Check sheet for the modelled part. Datum: model origin and axes. Units: mm. A direction names the side the tool comes from. Coordinates: 2 decimals unless noted, no trailing zeros. Write each loop counter-clockwise with the first axis right and the second up, starting at its lowest first coordinate (ties: lowest second). Pieces come first, ordered by that corner, then holes. Notation, with made-up numbers: M 89.25,73.5 L 140.25,73.5 A19 ccw 140.25,92.5 Z; hole C 34.5,61.5 d2. An arc over 180 degrees is marked long. Answer as CSV lines item,"result".
from build123d import *

# Parameters (mm, degrees)
SKETCH1_W               = 12
SKETCH1_H               = 88.272317903
SKETCH2_W               = 4.5
SKETCH2_H               = 60
CUT_EXTRUDE1_DEPTH      = 13
CUT_EXTRUDE1_DEPTH_BACK = 13
CUT_EXTRUDE2_DEPTH      = 5.5
CUT_EXTRUDE2_DEPTH_BACK = 20.5
SKETCH12_R              = 7.393886086
BOSS_EXTRUDE4_DEPTH     = 15
FILLET2_R               = 40
SKETCH4_R               = 6
CUT_EXTRUDE3_DEPTH      = 6
SKETCH5_R               = 2.25
CUT_EXTRUDE4_DEPTH      = 14.5
SKETCH6_R               = 7.5
BOSS_EXTRUDE1_DEPTH     = 13
SKETCH9_R               = 3.5
SKETCH10_R              = 9
BOSS_EXTRUDE2_DEPTH     = 8
SKETCH11_R              = 3.5
SKETCH11_R_2            = 2.25
BOSS_EXTRUDE3_DEPTH     = 0.5
FILLET1_R               = 0.5
SKETCH13_R              = 12
SKETCH13_R_2            = 3.5
BOSS_EXTRUDE5_DEPTH     = 17
FILLET3_R               = 16
SKETCH16_R              = 77.650275013
CUT_EXTRUDE5_DEPTH      = 22
SKETCH17_R              = 2
CUT_EXTRUDE6_DEPTH      = 22
CUT_EXTRUDE7_START      = -132.272318
SKETCH20_R              = 3.5
CUT_EXTRUDE7_DEPTH      = 132.272318
FILLET5_R               = 1


with BuildPart() as part:
    # Sketch1 → Revolve1 (revolve)
    with BuildSketch(Plane(origin=(0, 0, 0), x_dir=(0, 0, -1), z_dir=(1, 0, 0))):
        with Locations((-6, 44.136158952)):
            Rectangle(SKETCH1_W, SKETCH1_H)
    revolve(axis=Axis((0, 88.272317903, 0), (0, -1, 0)))

    # Sketch2 → Cut-Extrude1 (cut, two sides)
    with BuildSketch(Plane(origin=(0, 0, 0), x_dir=(0, 0, -1), z_dir=(1, 0, 0))) as cut_extrude1_sk:
        with Locations((-9.75, 30)):
            Rectangle(SKETCH2_W, SKETCH2_H)
        with Locations((9.75, 30)):
            Rectangle(SKETCH2_W, SKETCH2_H)
    extrude(amount=CUT_EXTRUDE1_DEPTH, mode=Mode.SUBTRACT)
    extrude(cut_extrude1_sk.sketch, amount=-CUT_EXTRUDE1_DEPTH_BACK, mode=Mode.SUBTRACT)

    # Sketch3 → Cut-Extrude2 (cut, two sides)
    with BuildSketch(Plane.XY.offset(7.5)) as cut_extrude2_sk:
        with BuildLine():
            Line((-12, 40), (-4.905482814, 4.032405892))
            ThreePointArc((-4.905482814, 4.032405892), (0, 0), (4.905482814, 4.032405892))
            Line((4.905482814, 4.032405892), (12, 40))
            Line((12, 40), (12, 0))
            Line((12, 0), (12, -1))
            Line((12, -1), (-12, -1))
            Line((-12, -1), (-12, 0))
            Line((-12, 0), (-12, 40))
        make_face()
    extrude(amount=CUT_EXTRUDE2_DEPTH, mode=Mode.SUBTRACT)
    extrude(cut_extrude2_sk.sketch, amount=-CUT_EXTRUDE2_DEPTH_BACK, mode=Mode.SUBTRACT)

    # Sketch12 → Boss-Extrude4 (add)
    with BuildSketch(Plane.XY.offset(7.5)):
        with Locations((0, 7.393886086)):
            Circle(SKETCH12_R)
    extrude(amount=-BOSS_EXTRUDE4_DEPTH)

    # Fillet2
    fillet2_edges = [part.edges().sort_by_distance(p)[0] for p in [
        (6.324137111, 11.224661628, 0),
        (-6.324137111, 11.224661628, 0),
    ]]
    fillet(fillet2_edges, radius=FILLET2_R)

    # Sketch4 → Cut-Extrude3 (cut)
    with BuildSketch(Plane.XY.offset(7.5)):
        with Locations((0, 5)):
            Circle(SKETCH4_R)
    extrude(amount=-CUT_EXTRUDE3_DEPTH, mode=Mode.SUBTRACT)

    # Sketch5 → Cut-Extrude4 (cut, through all)
    with BuildSketch(Plane.XY.offset(1.5)):
        with Locations((0, 5)):
            Circle(SKETCH5_R)
    extrude(amount=-CUT_EXTRUDE4_DEPTH, mode=Mode.SUBTRACT)

    # Sketch6 → Boss-Extrude1 (add, symmetric)
    with BuildSketch(Plane.XY):
        with Locations((0, 35)):
            Circle(SKETCH6_R)
    extrude(amount=BOSS_EXTRUDE1_DEPTH, both=True)

    # Sketch7 → Cut-Revolve1 (revolve, cut)
    with BuildSketch(Plane(origin=(0, 0, 0), x_dir=(0, 0, -1), z_dir=(1, 0, 0))):
        with BuildLine():
            Line((-7.5, 61.927405715), (-7.5, 51.927405715))
            Line((-7.5, 51.927405715), (-17.5, 51.927405715))
            ThreePointArc((-17.5, 51.927405715), (-24.571067812, 68.998473527), (-7.5, 61.927405715))
        make_face()
        with BuildLine():
            Line((7.5, 51.927405715), (17.5, 51.927405715))
            ThreePointArc((17.5, 51.927405715), (24.571067812, 68.998473527), (7.5, 61.927405715))
            Line((7.5, 61.927405715), (7.5, 51.927405715))
        make_face()
    revolve(axis=Axis((0, 35, 13), (0, 0, -1)), mode=Mode.SUBTRACT)

    # Cut-Sweep1: sweep along a path in Sketch8
    with BuildLine(Plane(origin=(0, 0, 0), x_dir=(0, 0, -1), z_dir=(1, 0, 0))) as cut_sweep1_path:
        Line((0, 88.272317903), (0, 25.420292636))
        ThreePointArc((0, 25.420292636), (3.646414893, 15.617430543), (12.812814028, 10.580608761))
    # Sketch9 → Cut-Sweep1 (sweep, cut)
    with BuildSketch(Plane(origin=(0, 88.272317903, 0), x_dir=(1, 0, 0), z_dir=(0, 1, 0))):
        Circle(SKETCH9_R)
    sweep(path=cut_sweep1_path.line, mode=Mode.SUBTRACT)

    # Sketch10 → Boss-Extrude2 (add, symmetric)
    with BuildSketch(Plane.XY):
        with Locations((0, 35)):
            Circle(SKETCH10_R)
    extrude(amount=BOSS_EXTRUDE2_DEPTH, both=True)

    # Sketch11 → Boss-Extrude3 (add)
    with BuildSketch(Plane.XY.offset(1.5)):
        with Locations((0, 5)):
            Circle(SKETCH11_R)
        with Locations((0, 5)):
            Circle(SKETCH11_R_2, mode=Mode.SUBTRACT)
    extrude(amount=BOSS_EXTRUDE3_DEPTH)

    # Fillet1
    fillet1_edges = [part.edges().sort_by_distance(p)[0] for p in [
        (-5.356920685, 2.297519515, 4.5),
        (5.356920685, 2.297519515, 4.5),
    ]]
    fillet(fillet1_edges, radius=FILLET1_R)

    # Sketch13 → Boss-Extrude5 (add)
    with BuildSketch(Plane(origin=(0, 88.272317903, 0), x_dir=(1, 0, 0), z_dir=(0, 1, 0))):
        Circle(SKETCH13_R)
        Circle(SKETCH13_R_2, mode=Mode.SUBTRACT)
    extrude(amount=BOSS_EXTRUDE5_DEPTH)

    # Sketch15 → Revolve2 (revolve)
    with BuildSketch(Plane(origin=(0, 0, 0), x_dir=(0, 0, -1), z_dir=(1, 0, 0))):
        Polygon((0, 105.272317903), (-40, 105.272317903), (-40, 115.272317903), (-11.5, 115.272317903), (-11.5, 116.272317903), (-10, 116.272317903), (-10, 123.272317903), (0, 123.272317903), align=None)
    revolve(axis=Axis((0, 88.826005803, 0), (0, -1, 0)))

    # Fillet3
    fillet3_edges = [part.edges().sort_by_distance(p)[0] for p in [
        (-12, 105.272317903, 0),
    ]]
    fillet(fillet3_edges, radius=FILLET3_R)

    # Sketch16 → Cut-Extrude5 (cut)
    with BuildSketch(Plane(origin=(0, 115.272317903, 0), x_dir=(1, 0, 0), z_dir=(0, 1, 0))):
        Circle(SKETCH16_R)
        with BuildLine():
            Line((-30.638590038, -17.23454387), (30.638590038, -17.23454387))
            ThreePointArc((30.638590038, -17.23454387), (38.298237548, -11.543179837), (35.059424473, -2.566993877))
            Line((35.059424473, -2.566993877), (9.523883126, 14.364022856))
            ThreePointArc((9.523883126, 14.364022856), (0, 17.23454387), (-9.523883126, 14.364022856))
            Line((-9.523883126, 14.364022856), (-35.059424473, -2.566993877))
            ThreePointArc((-35.059424473, -2.566993877), (-38.298237548, -11.543179837), (-30.638590038, -17.23454387))
        make_face(mode=Mode.SUBTRACT)
    extrude(amount=-CUT_EXTRUDE5_DEPTH, mode=Mode.SUBTRACT)

    # Sketch17 → Cut-Extrude6 (cut)
    with BuildSketch(Plane(origin=(0, 115.272317903, 0), x_dir=(1, 0, 0), z_dir=(0, 1, 0))):
        with Locations((-30.638590038, -9.23454387)):
            Circle(SKETCH17_R)
        with Locations((30.638590038, -9.23454387)):
            Circle(SKETCH17_R)
    extrude(amount=-CUT_EXTRUDE6_DEPTH, mode=Mode.SUBTRACT)

    # Sketch19 → Revolve3 (revolve)
    with BuildSketch(Plane.XY):
        Polygon((-10, 123.272317903), (-9, 153.272317903), (-7.5, 153.272317903), (-7.5, 158.272317903), (0, 158.272317903), (0, 123.272317903), align=None)
    revolve(axis=Axis((0, 123.272317903, 0), (0, 1, 0)))

    # Sketch20 → Cut-Extrude7 (cut)
    with BuildSketch(Plane(origin=(0, 158.272317903, 0), x_dir=(1, 0, 0), z_dir=(0, 1, 0)).offset(CUT_EXTRUDE7_START)):
        Circle(SKETCH20_R)
    extrude(amount=CUT_EXTRUDE7_DEPTH, mode=Mode.SUBTRACT)

    # Fillet5
    fillet5_edges = [part.edges().sort_by_distance(p)[0] for p in [
        (-3.5, 158.272317903, 0),
    ]]
    fillet(fillet5_edges, radius=FILLET5_R)


solid = part.part
1) Tool access check on faces 1 (the face through (-1.172, 43.923, -7.746)), 2 (the face through (0.7, 2.7, 2)), 3 (the face through (-11.4, 115.8, -1.5)), 4 (the face through (-32.3, 105.272, 7.7)). Record the directions out of +Z, -Z, +X, -X, +Y, -Y that give a thin tool (end or side, any length) a straight path to the whole face; none if there is none.
Answer key:
face 1,"-Z"
face 2,"+Z, -Y"
face 3,"+Y"
face 4,"+Z, -X, -Y"
2) Thickness scan on line 1 along Y through (x, z) = (0, 1.85); line 2 along Y through (x, z) = (0, -4.5); line 3 along Y through (x, z) = (-28, 4). Record the ranges inside material, lowest first.
Answer key:
line 1,"y = 1.5 to 2.75, 7.25 to 8.5, 11 to 17.78"
line 2,"y = 0 to 2.75, 7.25 to 10.19, 20.73 to 158.27"
line 3,"y = 105.27 to 115.27"
3) Depth check by flat-ended pin: P1, Ø12, axis at x = -27.5, y = 117, coming from the -Z side; P2, Ø15, axis at x = -2.5, y = 32, coming from the -Z side; P3, Ø3.5, axis at x = 0, y = 5, coming from the +Z side; P4, Ø6, axis at y = 130, z = -8, coming from the +X side. Enter the tip coordinate at first touch or a pass-through.
Answer key:
P1,"stops at z = -6.25"
P2,"stops at z = -13"
P3,"passes through"
P4,"stops at x = 8.4"
4) Mould release check, pull along Z, two halves, no side actions. Record for faces 5 (the face through (22.47, 109.86, -5.78)), 6 (the face through (7.244, 13.713, 0.105)), 7 (the face through (29.05, 110.34, 10.45)): pulls with the +Z half, pulls with the -Z half, needs draft (parallel to the pull), parting line crosses it, or undercut.
Answer key:
face 5,"pulls with the -Z half"
face 6,"needs draft"
face 7,"undercut"
5) Section check A-A, the plane y = 50. Record the boundary of the cut face in (x, z).
Answer key:
outline,"M -9.37,-7.5 L 9.37,-7.5 A12 ccw 9.37,7.5 L -9.37,7.5 A12 ccw Z; hole C 0,0 d7"
6) Section check B-B, the plane y = 110.5. Record the boundary of the cut face in (x, z).
Answer key:
outline,"M -35.06,2.57 L -9.52,-14.36 A17.23 ccw 9.52,-14.36 L 35.06,2.57 A8 ccw 30.64,17.23 L -30.64,17.23 A8 ccw Z; hole C -30.64,9.23 d4; hole C 0,0 d7; hole C 30.64,9.23 d4"
7) Section check C-C, the plane z = -6. Give the number of separate pieces and of enclosed holes in the cut face, plus the area to 3 significant figures.
Answer key:
separate pieces,"1"
enclosed holes,"2"
area,"3,130 mm2"
